Geometry: final body of the model. Coordinates: model frame, mm. Give positions to 0.01 mm unless a question says otherwise; leave off trailing zeros. Loops run counter-clockwise (first coordinate to the right, second up) from the corner with the lowest first, then second, coordinate; pieces in that order, holes last.
from build123d import *

# Parameters (mm, degrees)
ESQUISSE1_R                               = 55
ESQUISSE1_R_2                             = 17
BOSS_EXTRU_1_DEPTH                        = 5
TROU_POUR_TARAUDAGE_POUR_TROU_TARAUD_M8_D = 6.8
TROU_POUR_TARAUDAGE_POUR_TROU_TARAUD_M6_D = 5


with BuildPart() as part:
    # Esquisse1 → Boss.-Extru.1 (new body)
    with BuildSketch(Plane.XY):
        Circle(ESQUISSE1_R)
        Circle(ESQUISSE1_R_2, mode=Mode.SUBTRACT)
    extrude(amount=BOSS_EXTRU_1_DEPTH)

    # Trou pour taraudage pour trou taraudé M8x1.252 (through all)
    with Locations(Plane.XY.offset(5)):
        with Locations((0, 45), (45, 0), (0, -45), (-45, 0)):
            Hole(TROU_POUR_TARAUDAGE_POUR_TROU_TARAUD_M8_D / 2)

    # Trou pour taraudage pour trou taraudé M6x1.02 (through all)
    with Locations(Plane.XY.offset(5)):
        with Locations((11, 19.052558883), (22, 0), (11, -19.052558883), (-11, -19.052558883), (-22, 0), (-11, 19.052558883)):
            Hole(TROU_POUR_TARAUDAGE_POUR_TROU_TARAUD_M6_D / 2)


solid = part.part
Item 1: Section query D-D on y = -13. Return loops of the section in (x, z), plus the area to 3 significant figures.
Values follow:
outline: (-53.44, 0) - (-10.95, 0) - (-10.95, 5) - (-53.44, 5) - close; (10.95, 0) - (53.44, 0) - (53.44, 5) - (10.95, 5) - close
area: 425 mm2
Item 2: Section query C-C on z = 1.4. Give the number of separate pieces and of enclosed holes in the cut face, plus the area to 3 significant figures.
Values follow:
separate pieces: 1
enclosed holes: 11
area: 8,330 mm2
Item 3: Section query A-A on x = 0. Return loops of the section in (y, z), plus the area to 3 significant figures.
Values follow:
outline: (-55, 0) - (-48.4, 0) - (-48.4, 5) - (-55, 5) - close; (-41.6, 0) - (-17, 0) - (-17, 5) - (-41.6, 5) - close; (17, 0) - (41.6, 0) - (41.6, 5) - (17, 5) - close; (48.4, 0) - (55, 0) - (55, 5) - (48.4, 5) - close
area: 312 mm2
Item 4: Ray query, probe 1 along Y at (x, z) = (0, 1.15); probe 2 along X at (y, z) = (-20, 4.5); probe 3 along Y at (x, z) = (45, 2.5). Return the intervals inside material, ascending.
Values follow:
probe 1: y = -55 to -48.4, -41.6 to -17, 17 to 41.6, 48.4 to 55
probe 2: x = -51.23 to -13.31, -8.69 to 8.69, 13.31 to 51.23
probe 3: y = -31.62 to -3.4, 3.4 to 31.62
Item 5: Pin query (flat end, axial travel): pin 1 (2 mm diameter, centred on x = 8.5, z = 2, fed in from -Y); pin 2 (3 mm diameter, centred on x = 2.5, z = 2.5, fed in from -Y). Return the tip coordinate at first contact, or that it passes through.
Values follow:
pin 1: stops at y = -54.49
pin 2: stops at y = -54.99
Item 6: Section query B-B on y = 0. Return loops of the section in (x, z).
Values follow:
outline: (-55, 0) - (-48.4, 0) - (-48.4, 5) - (-55, 5) - close; (-41.6, 0) - (-24.5, 0) - (-24.5, 5) - (-41.6, 5) - close; (-19.5, 0) - (-17, 0) - (-17, 5) - (-19.5, 5) - close; (17, 0) - (19.5, 0) - (19.5, 5) - (17, 5) - close; (24.5, 0) - (41.6, 0) - (41.6, 5) - (24.5, 5) - close; (48.4, 0) - (55, 0) - (55, 5) - (48.4, 5) - close
Item 7: Draft query along X for faces 1 (the face through (-48.14, -1.3, 2.47)), 2 (the face through (-13, -11.5, 0)), 3 (the face through (-10.675, -16.574, 2.465)), 4 (the face through (-11.923, -53.692, 2.465)). Return one class per face: +X half, -X half, draft (parallel to the pull), parting line (faces both ways), or undercut.
Values follow:
face 1: undercut
face 2: draft
face 3: undercut
face 4: parting line
